Check sheet for the modelled part. Datum: model origin and axes. Units: mm. Face numbers are marked on the shaded views. A direction names the side the tool comes from. Round coordinates to 2 decimals unless told otherwise and drop trailing zeros. Order: outer loops, then holes, each group sorted by start corner. A loop starts at its lowest first (then second) coordinate and runs counter-clockwise, first axis right, second up.
```python
from build123d import *

# Parameters (mm, degrees)
F1_DEPTH  = 32
F2_DEPTH  = 12.5
F4_DEPTH  = 19
F5_R      = 10
F6_R      = 5
F7_DEPTH  = 19
F6_R_2    = 19.5
F8_DEPTH  = 12
F10_DEPTH = 6
F11_W     = 22
F11_H     = 56
F12_DEPTH = 6
F14_DEPTH = 70
F15_R     = 7.5
F16_DEPTH = 70


with BuildPart() as f1:
    # F0 (on Front) → F1 (new body, symmetric)
    with BuildSketch(Plane.XZ):
        Polygon((-45, 77.9422863406), (0, 0), (140, 0), (140, 19), (125, 19), (55, 19), (10.9696551146, 19), (-19.0455173281, 70.9878036687), (25.1217782649, 96.4878036687), (15.6217782649, 112.9422863406), align=None)
    extrude(amount=F1_DEPTH, both=True)

    # F0 (on Front) → F2 (join, symmetric)
    with BuildSketch(Plane.XZ):
        Polygon((55, 19), (125, 19), (125, 59), (110, 59), (110, 26), (70, 26), (70, 59), (55, 59), align=None)
    extrude(amount=F2_DEPTH, both=True)

    # F3 (on face) → F4 (cut, through all)
    with BuildSketch(Plane(origin=(-45, 0, 77.9422863406), x_dir=(0.8660254038, 0, 0.5), z_dir=(-0.5, 0, 0.8660254038))):
        with BuildLine():
            ThreePointArc((38, 32), (60.627416998, 22.627416998), (70, 0))
            Line((70, 0), (70, 32))
            Line((70, 32), (38, 32))
        make_face()
        with BuildLine():
            Line((70, -32), (70, 0))
            ThreePointArc((70, 0), (60.627416998, -22.627416998), (38, -32))
            Line((38, -32), (70, -32))
        make_face()
    extrude(amount=-F4_DEPTH, mode=Mode.SUBTRACT)

    # F5
    f5_edges = [f1.edges().sort_by_distance(p)[0] for p in [
        (10.969655, 0, 19),
    ]]
    fillet(f5_edges, radius=F5_R)

    # F6 (on face) → F7 (cut, through all)
    with BuildSketch(Plane(origin=(-45, 0, 77.9422863406), x_dir=(0.8660254038, 0, 0.5), z_dir=(-0.5, 0, 0.8660254038))):
        with Locations((38, 0)):
            Circle(F6_R)
    extrude(amount=-F7_DEPTH, mode=Mode.SUBTRACT)

    # F6 (on face) → F8 (cut)
    with BuildSketch(Plane(origin=(-45, 0, 77.9422863406), x_dir=(0.8660254038, 0, 0.5), z_dir=(-0.5, 0, 0.8660254038))):
        with Locations((38, 0)):
            Circle(F6_R_2)
        with Locations((38, 0)):
            Circle(F6_R, mode=Mode.SUBTRACT)
    extrude(amount=-F8_DEPTH, mode=Mode.SUBTRACT)

    # F9 (on face) → F10 (cut)
    with BuildSketch(Plane(origin=(-45, 0, 77.9422863406), x_dir=(0.8660254038, 0, 0.5), z_dir=(-0.5, 0, 0.8660254038))):
        with BuildLine():
            Line((21.8987578119, 11), (0, 11))
            Line((0, 11), (0, -11))
            Line((0, -11), (21.8987578119, -11))
            ThreePointArc((21.8987578119, -11), (18.5, 0), (21.8987578119, 11))
        make_face()
        with BuildLine():
            Line((68.0499584026, 11), (54.1012421881, 11))
            ThreePointArc((54.1012421881, 11), (56.630944993, 5.7565518035), (57.5, 0))
            ThreePointArc((57.5, 0), (56.630944993, -5.7565518035), (54.1012421881, -11))
            Line((54.1012421881, -11), (68.0499584026, -11))
            ThreePointArc((68.0499584026, -11), (70, 0), (68.0499584026, 11))
        make_face()
    extrude(amount=-F10_DEPTH, mode=Mode.SUBTRACT)

    # F11 (on face) → F12 (cut)
    with BuildSketch(Plane(origin=(0, 0, 0), x_dir=(0, -1, 0), z_dir=(-0.8660254038, 0, -0.5))):
        with Locations((0, 56)):
            Rectangle(F11_W, F11_H)
    extrude(amount=-F12_DEPTH, mode=Mode.SUBTRACT)

    # F13 (on face) → F14 (cut, through all)
    with BuildSketch(Plane.YZ.offset(125)):
        with BuildLine():
            ThreePointArc((-12.5, 46.5), (-8.8388347372, 55.3388347924), (7.81e-08, 59))
            Line((7.81e-08, 59), (-12.5, 59))
            Line((-12.5, 59), (-12.5, 46.5))
        make_face()
        with BuildLine():
            ThreePointArc((7.81e-08, 59), (8.8388347924, 55.3388347372), (12.5, 46.5))
            Line((12.5, 46.5), (12.5, 59))
            Line((12.5, 59), (7.81e-08, 59))
        make_face()
    extrude(amount=-F14_DEPTH, mode=Mode.SUBTRACT)

    # F15 (on face) → F16 (cut, through all)
    with BuildSketch(Plane.YZ.offset(125)):
        with Locations((0, 46.5)):
            Circle(F15_R)
    extrude(amount=-F16_DEPTH, mode=Mode.SUBTRACT)


solid = f1.part
```
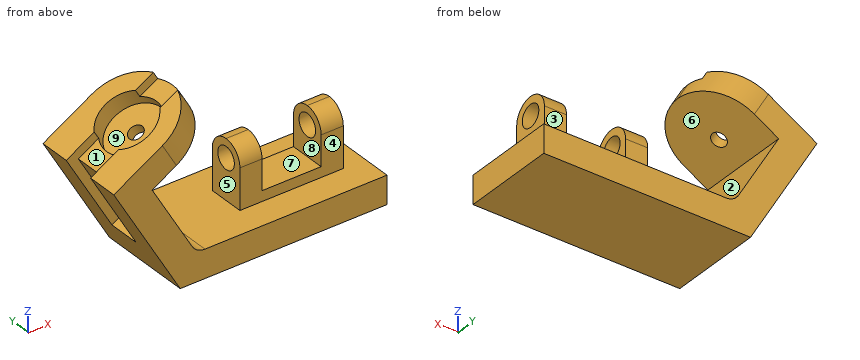
Item 1: Sectioned sample at C-C (y = 15). Record the cut outline in (x, z), and give its area (3 significant figures).
Answer:
outline: (-45, 77.94) - (0, 0) - (140, 0) - (140, 19) - (16.74, 19) arc R10 cw to (8.08, 24) - (-19.05, 70.99) - (21.89, 94.62) - (12.39, 111.08) - (-1.3, 103.17) - (4.7, 92.78) - (-16.88, 80.32) - (-22.88, 90.71) - close
area: 4,770 mm2
Item 2: Sectioned sample at A-A (x = 63). Record the cut outline in (y, z).
Answer:
outline: (-32, 0) - (32, 0) - (32, 19) - (12.5, 19) - (12.5, 46.5) arc R12.5 ccw to (-12.5, 46.5) - (-12.5, 19) - (-32, 19) - close; hole circle Ø15 at (0, 46.5)
Item 3: Go/stop test with flat-tipped pins: P1, Ø7.5, axis at y = -4.5, z = 38.5, coming from the -X side; P2, Ø3, axis at x = 107, y = -23, coming from the +Z side; P3, Ø12, axis at y = 0, z = 46.5, coming from the +X side. Record where each tip stops, or that it passes through.
Answer:
P1: stops at x = -17.46
P2: stops at z = 19
P3: stops at x = -1.44
Item 4: Scan lines: line 1 along Y through (x, z) = (115, 46); line 2 along Z through (x, y) = (74, 14); line 3 along X through (y, z) = (-13.5, 97.5). Record each from-to range of solid material in increasing order.
Answer:
line 1: y = -12.5 to -7.48, 7.48 to 12.5
line 2: z = 0 to 19
line 3: x = 3.84 to 21.09
Item 5: Release check for a two-part mould opening along Z. For the marked faces 6, 7, 8 and 9 record: released by +Z, released by -Z, zero draft, split by the parting line, or undercut.
Answer:
face 6: undercut
face 7: released by +Z
face 8: zero draft
face 9: undercut
Item 6: Sectioned sample at D-D (x = -32). Record the cut outline in (y, z).
Answer:
outline: (-32, 55.43) - (-11, 55.43) - (-11, 67.43) - (11, 67.43) - (11, 55.43) - (32, 55.43) - (32, 85.45) - (11, 85.45) - (11, 78.52) - (-11, 78.52) - (-11, 85.45) - (-32, 85.45) - close
Item 7: Sectioned sample at B-B (z = 50.5). Record the cut outline in (x, y), and give its area (3 significant figures).
Answer:
outline: (-29.16, -32) - (-7.22, -32) - (-7.22, 32) - (-29.16, 32) - (-29.16, 11) - (-22.23, 11) - (-22.23, -11) - (-29.16, -11) - close; (55, -11.84) - (70, -11.84) - (70, -6.34) - (55, -6.34) - close; (55, 6.34) - (70, 6.34) - (70, 11.84) - (55, 11.84) - close; (110, -11.84) - (125, -11.84) - (125, -6.34) - (110, -6.34) - close; (110, 6.34) - (125, 6.34) - (125, 11.84) - (110, 11.84) - close
area: 1,580 mm2
Item 8: Access from +Z, -Z, +X, -X, +Y, -Y to the whole of each face (thin tool, end or side, straight path). Record for the marked faces 1, 2, 3, 4 and 5.
Answer:
face 1: +Z, -X
face 2: +Y, -Y
face 3: +Z, +X, +Y
face 4: +Z, +X, -Y
face 5: +Z, +Y, -Y
